```python
from build123d import *

# Parameters (mm, degrees)
EXTRUDE_1_DEPTH          = 12
SKETCH_2_R               = 6
EXTRUDE_2_DEPTH          = 30
SKETCH_3_R               = 3
CUT_EXTRUDE_1_DEPTH      = 103.282410285
SKETCH_5_R               = 5
CUT_EXTRUDE_2_DEPTH      = 81.274528962
CUT_EXTRUDE_3_DEPTH      = 81.274528962
PATTERN_CIRCULAR_2_COUNT = 3
SKETCH_7_R               = 3
CUT_EXTRUDE_4_DEPTH      = 100.361803703
SKETCH_8_R               = 3
CUT_EXTRUDE_5_DEPTH      = 96.764127078


with BuildPart() as part:
    # 草图1 → 凸台-拉伸1 (new body)
    with BuildSketch(Plane.XY):
        Polygon((0, 60), (-51.961524227, -30), (51.961524227, -30), align=None)
    extrude(amount=EXTRUDE_1_DEPTH)

    # 草图2 → 凸台-拉伸2 (add, symmetric)
    with BuildSketch(Plane(origin=(0, 0, 0), x_dir=(0, 0, -1), z_dir=(1, 0, 0))):
        with Locations((-6, -36)):
            Circle(SKETCH_2_R)
        with BuildLine():
            ThreePointArc((-6, -30), (-1.757359313, -31.757359313), (0, -36))
            Line((0, -36), (0, -30))
            Line((0, -30), (-6, -30))
        make_face()
        with BuildLine():
            Line((-12, -30), (-12, -36))
            ThreePointArc((-12, -36), (-10.242640687, -31.757359313), (-6, -30))
            Line((-6, -30), (-12, -30))
        make_face()
    extrude_2 = extrude(amount=EXTRUDE_2_DEPTH, both=True)

    # 草图3 → 切除-拉伸1 (cut, through all)
    with BuildSketch(Plane(origin=(30, 0, 0), x_dir=(0, 0, -1), z_dir=(1, 0, 0))):
        with Locations((-6, -36)):
            Circle(SKETCH_3_R)
    extrude(amount=-CUT_EXTRUDE_1_DEPTH, mode=Mode.SUBTRACT)

    # 草图5 → 切除-拉伸2 (cut, through all)
    with BuildSketch(Plane(origin=(0, 0, 0), x_dir=(-1, 0, 0), z_dir=(0, 0, -1))):
        Circle(SKETCH_5_R)
    extrude(amount=-CUT_EXTRUDE_2_DEPTH, mode=Mode.SUBTRACT)

    # 草图6 → 切除-拉伸3 (cut, through all)
    with BuildSketch(Plane(origin=(0, 0, 0), x_dir=(-1, 0, 0), z_dir=(0, 0, -1))):
        Polygon((-30, -30), (-51.961524227, -30), (-40.980762114, -10.980762114), align=None)
        Polygon((10.980762114, 40.980762114), (-10.980762114, 40.980762114), (0, 60), align=None)
        Polygon((30, -30), (40.980762114, -10.980762114), (51.961524227, -30), align=None)
    extrude(amount=-CUT_EXTRUDE_3_DEPTH, mode=Mode.SUBTRACT)

    # 阵列(圆周)2: 凸台-拉伸2 ×3 about axis
    pattern_circular_2_axis = Axis((0, 0, 0), (0, 0, 1))
    for i in range(1, PATTERN_CIRCULAR_2_COUNT):
        add(extrude_2.rotate(pattern_circular_2_axis, i * 360 / PATTERN_CIRCULAR_2_COUNT))

    # 草图7 → 切除-拉伸4 (cut, through all)
    with BuildSketch(Plane(origin=(15, -25.980762114, 0), x_dir=(0.8660254037844434, 0.49999999999999195, 0), z_dir=(0.49999999999999195, -0.8660254037844434, 0))):
        with Locations((36, 6)):
            Circle(SKETCH_7_R)
    extrude(amount=-CUT_EXTRUDE_4_DEPTH, mode=Mode.SUBTRACT)

    # 草图8 → 切除-拉伸5 (cut, through all)
    with BuildSketch(Plane(origin=(15, 25.980762114, 0), x_dir=(0.8660254037844363, -0.5000000000000043, 0), z_dir=(0.5000000000000042, 0.8660254037844362, 0))):
        with Locations(Location((-36, -6, 0), (0, 0, 180))):
            Circle(SKETCH_8_R)
    extrude(amount=-CUT_EXTRUDE_5_DEPTH, mode=Mode.SUBTRACT)


solid = part.part
```
Could you check a few things on this model? Use its own coordinates, in mm. A direction names the side the tool comes from. Coordinates: 2 decimals unless noted, no trailing zeros. Write each loop counter-clockwise with the first axis right and the second up, starting at its lowest first coordinate (ties: lowest second). Pieces come first, ordered by that corner, then holes. Notation, with made-up numbers: (84, 83) -> (107, 83) arc R10 ccw to (107, 88) -> close; hole circle Ø4 at (20.25, -26). An arc over 180 degrees is marked (long way). Return JSON: item names as keys, results as strings.
(1) We'd pull the mould along Z, two halves only. Please class faces 4 (the flat face through (-2, -12, 12)), 5 (the flat face through (35.567, -20.357, 5.916)), 6 (the cylindrical face through (0, -33, 6)): +Z half, -Z half, draft (parallel to the pull), parting line (faces both ways), or undercut.
Numbers:
{"face 4": "+Z half", "face 5": "draft", "face 6": "undercut"}
(2) Imagine slicing it at A-A, the plane x = 0. Please give me the cut outline in (y, z).
Numbers:
{"outline": "(-36, 0) -> (-5, 0) -> (-5, 12) -> (-36, 12) arc R6 ccw to start; (5, 0) -> (40.98, 0) -> (40.98, 12) -> (5, 12) -> close; hole circle Ø6 at (-36, 6)"}
(3) Imagine slicing it at B-B, the plane z = 7.5. Please give me the cut outline in (x, y), then the cut area to 3 significant figures.
Numbers:
{"outline": "(-51.21, -5.08) -> (-48.43, -6.68) -> (-18.43, 45.28) -> (-21.21, 46.89) -> close; (-43.93, -9.28) -> (-40.98, -10.98) -> (-30, -30) -> (-30, -33.4) -> (30, -33.4) -> (30, -30) -> (40.98, -10.98) -> (43.93, -9.28) -> (13.93, 42.68) -> (10.98, 40.98) -> (-10.98, 40.98) -> (-13.93, 42.68) -> close; (-30, -41.81) -> (30, -41.81) -> (30, -38.6) -> (-30, -38.6) -> close; (18.43, 45.28) -> (48.43, -6.68) -> (51.21, -5.08) -> (21.21, 46.89) -> close; hole circle Ø10 at (0, 0)", "area": "5,160 mm2"}
(4) Imagine slicing it at C-C, the plane y = 0. Count the separate pieces of the cut face and the enclosed holes in it, then the cut area to 3 significant figures.
Numbers:
{"separate pieces": "2", "enclosed holes": "2", "area": "943 mm2"}
(5) I'm going to push flat-ended pins straight in: pin 1 (6 mm diameter, centred on x = 0, y = 0, fed in from -Z); pin 2 (6 mm diameter, centred on x = -32, z = 4, fed in from +Y); pin 3 (3 mm diameter, centred on y = 2, z = 6, fed in from +X); pin 4 (5 mm diameter, centred on x = 36, z = 2, fed in from +Y). Where does each tip first touch, or does it pass through?
Numbers:
{"pin 1": "passes through", "pin 2": "stops at y = 33.34", "pin 3": "stops at x = 48.21", "pin 4": "stops at y = 24.06"}
(6) Imagine slicing it at D-D, the plane z = 1.75. Please give me the cut outline in (x, y), then the cut area to 3 significant figures.
Numbers:
{"outline": "(-49.84, -5.86) -> (-40.98, -10.98) -> (-30, -30) -> (-30, -40.24) -> (30, -40.24) -> (30, -30) -> (40.98, -10.98) -> (49.84, -5.86) -> (19.84, 46.1) -> (10.98, 40.98) -> (-10.98, 40.98) -> (-19.84, 46.1) -> close; hole circle Ø10 at (0, 0)", "area": "5,810 mm2"}
(7) I need wall thicknesses on L1, parallel to Y at x = -27, z = 4; L2, parallel to Y at x = 0, z = 8.25; L3, parallel to X at y = 20, z = 3.5. Which ranges of each line are inside material? Lowest first, please.
Numbers:
{"L1": "y = -41.66 to -38.24, -33.76 to 20.76, 29.71 to 36.55", "L2": "y = -41.56 to -37.98, -34.02 to -5, 5 to 40.98", "L3": "x = -36.32 to -31.94, -28.11 to 28.11, 31.94 to 36.32"}
(8) Which directions (+Z, -Z, +X, -X, +Y, -Y) give clear straight access to the entire face, cutting with the end or side of a thin tool? Please do faces 1 (the flat face through (13.795, 42.605, 8.751)), 2 (the flat face through (-30, -33, 7)), 3 (the flat face through (30, -33, 7)).
Numbers:
{"face 1": "+Z, -Z, +Y", "face 2": "+Z, -Z, -X, -Y", "face 3": "+Z, -Z, +X, -Y"}
